```python
from build123d import *

# Parameters (mm, degrees)
PAD017_DEPTH                  = 15.3
PAD017_MIRRORED033_2_DEPTH    = 15.3
PAD023_DEPTH                  = 2
PAD023_MIRRORED043_2_DEPTH    = 2
SKETCH061_R                   = 1
PAD019_DEPTH                  = 4
POCKET060_DEPTH               = 6
POCKET060_MIRRORED038_2_DEPTH = 6
PAD020_DEPTH                  = 30
POCKET068_DEPTH               = 20
CHAMFER034_SIZE               = 1
CHAMFER026_SIZE               = 1
CHAMFER029_SIZE               = 0.5
CHAMFER028_SIZE               = 0.5
CHAMFER033_SIZE               = 0.5
POCKET063_DEPTH               = 5
SKETCH082_W                   = 9.4
SKETCH082_H                   = 50
POCKET066_DEPTH               = 5
POCKET053_DEPTH               = 10
POCKET065_DEPTH               = 10
POCKET052_DEPTH               = 10
POCKET056_DEPTH               = 10
POCKET057_DEPTH               = 10
POCKET071_DEPTH               = 10
SKETCH072_R                   = 2
POCKET072_DEPTH               = 5
CHAMFER031_SIZE               = 1.5


with BuildPart() as part:
    # Sketch076 → Pad017 (new body)
    with BuildSketch(Plane.XY):
        with BuildLine():
            ThreePointArc((-47.2, 25.2), (-49.32132, 24.32132), (-50.2, 22.2))
            Line((-50.2, 22.2), (-50.2, 0))
            Line((-52.2, 0), (-50.2, 0))
            Line((-52.2, 22.2), (-52.2, 0))
            ThreePointArc((-47.2, 27.2), (-50.735534, 25.735534), (-52.2, 22.2))
            Line((-47.2, 27.2), (0, 27.2))
            Line((0, 27.2), (0, 25.2))
            Line((-47.2, 25.2), (0, 25.2))
        make_face()
    pad017 = extrude(amount=PAD017_DEPTH)

    # Sketch076 Mirrored033 2 → Pad017 Mirrored033 2 (add)
    with BuildSketch(Plane(origin=(0, 0, 0), x_dir=(-1, 0, 0), z_dir=(0, 0, -1))):
        with BuildLine():
            ThreePointArc((-47.2, 25.2), (-49.32132, 24.32132), (-50.2, 22.2))
            Line((-50.2, 22.2), (-50.2, 0))
            Line((-52.2, 0), (-50.2, 0))
            Line((-52.2, 22.2), (-52.2, 0))
            ThreePointArc((-47.2, 27.2), (-50.735534, 25.735534), (-52.2, 22.2))
            Line((-47.2, 27.2), (0, 27.2))
            Line((0, 27.2), (0, 25.2))
            Line((-47.2, 25.2), (0, 25.2))
        make_face()
    pad017_mirrored033_2 = extrude(amount=-PAD017_MIRRORED033_2_DEPTH)

    # Mirrored031: Pad017, Pad017 Mirrored033 2 across Sketch076 H_Axis
    add(pad017.mirror(Plane.ZX))
    add(pad017_mirrored033_2.mirror(Plane.ZX))

    # Sketch074 → Pad023 (join)
    with BuildSketch(Plane.XY):
        with BuildLine():
            ThreePointArc((-47.2, 25.2), (-49.32132, 24.32132), (-50.2, 22.2))
            Line((-50.2, 22.2), (-50.2, 0))
            Line((-50.2, 0), (0, 0))
            Line((0, 0), (0, 25.2))
            Line((-47.2, 25.2), (0, 25.2))
        make_face()
    pad023 = extrude(amount=PAD023_DEPTH)

    # Sketch074 Mirrored043 2 → Pad023 Mirrored043 2 (add)
    with BuildSketch(Plane(origin=(0, 0, 0), x_dir=(-1, 0, 0), z_dir=(0, 0, -1))):
        with BuildLine():
            ThreePointArc((-47.2, 25.2), (-49.32132, 24.32132), (-50.2, 22.2))
            Line((-50.2, 22.2), (-50.2, 0))
            Line((-50.2, 0), (0, 0))
            Line((0, 0), (0, 25.2))
            Line((-47.2, 25.2), (0, 25.2))
        make_face()
    pad023_mirrored043_2 = extrude(amount=-PAD023_MIRRORED043_2_DEPTH)

    # Mirrored037: Pad023, Pad023 Mirrored043 2 across Sketch074 H_Axis
    add(pad023.mirror(Plane.ZX))
    add(pad023_mirrored043_2.mirror(Plane.ZX))

    # Sketch061 (on Face19 of MultiTransform012) → Pad019 (join)
    with BuildSketch(Plane.XY.offset(2)):
        with BuildLine():
            ThreePointArc((50.2, 22.2), (49.32132, 24.32132), (47.2, 25.2))
            Line((47.2, 25.2), (44, 25.2))
            Line((44, 22), (44, 25.2))
            ThreePointArc((44, 22), (44.87868, 19.87868), (47, 19))
            Line((47, 19), (50.2, 19))
            Line((50.2, 22.2), (50.2, 19))
        make_face()
        with Locations((47, 22)):
            Circle(SKETCH061_R, mode=Mode.SUBTRACT)
        with BuildLine():
            ThreePointArc((-41, 22), (-38, 19), (-35, 22))
            Line((-35, 22), (-35, 25.2))
            Line((-41, 25.2), (-35, 25.2))
            Line((-41, 22), (-41, 25.2))
        make_face()
        with Locations((-38, 22)):
            Circle(SKETCH061_R, mode=Mode.SUBTRACT)
    pad019 = extrude(amount=PAD019_DEPTH)

    # Mirrored035: Pad019 across Sketch061 H_Axis
    add(pad019.mirror(Plane(origin=(0, 0, 2), x_dir=(0, 0, 1), z_dir=(0, 1, 0))))

    # Sketch068 (on Face5 of Mirrored035) → Pocket060 (cut)
    with BuildSketch(Plane.XY.offset(15.3)):
        with BuildLine():
            ThreePointArc((-47.2, 27.2), (-50.735534, 25.735534), (-52.2, 22.2))
            Line((-52.2, 0), (-52.2, 22.2))
            Line((-51.1, 0), (-52.2, 0))
            Line((-51.1, 22.2), (-51.1, 0))
            ThreePointArc((-47.2, 26.1), (-49.957716, 24.957716), (-51.1, 22.2))
            Line((0, 26.1), (-47.2, 26.1))
            Line((0, 27.2), (0, 26.1))
            Line((-47.2, 27.2), (0, 27.2))
        make_face()
    pocket060 = extrude(amount=-POCKET060_DEPTH, mode=Mode.SUBTRACT)

    # Sketch068 Mirrored038 2 → Pocket060 Mirrored038 2 (cut)
    with BuildSketch(Plane(origin=(0, 0, 15.3), x_dir=(-1, 0, 0), z_dir=(0, 0, -1))):
        with BuildLine():
            ThreePointArc((-47.2, 27.2), (-50.735534, 25.735534), (-52.2, 22.2))
            Line((-52.2, 0), (-52.2, 22.2))
            Line((-51.1, 0), (-52.2, 0))
            Line((-51.1, 22.2), (-51.1, 0))
            ThreePointArc((-47.2, 26.1), (-49.957716, 24.957716), (-51.1, 22.2))
            Line((0, 26.1), (-47.2, 26.1))
            Line((0, 27.2), (0, 26.1))
            Line((-47.2, 27.2), (0, 27.2))
        make_face()
    pocket060_mirrored038_2 = extrude(amount=POCKET060_MIRRORED038_2_DEPTH, mode=Mode.SUBTRACT)

    # Mirrored042: Pocket060, Pocket060 Mirrored038 2 across Sketch068 H_Axis
    add(pocket060.mirror(Plane(origin=(0, 0, 15.3), x_dir=(0, 0, 1), z_dir=(0, 1, 0))), mode=Mode.SUBTRACT)
    add(pocket060_mirrored038_2.mirror(Plane(origin=(0, 0, 15.3), x_dir=(0, 0, 1), z_dir=(0, 1, 0))), mode=Mode.SUBTRACT)

    # Sketch060 → Pad020 (join, symmetric)
    with BuildSketch(Plane.YZ):
        with BuildLine():
            ThreePointArc((-26.1, 12.9), (-26.7, 12.3), (-26.1, 11.7))
            Line((-26.1, 12.9), (-26.1, 11.7))
        make_face()
    pad020 = extrude(amount=PAD020_DEPTH, both=True)

    # Sketch060 → Pocket068 (cut, symmetric)
    with BuildSketch(Plane.YZ):
        with BuildLine():
            ThreePointArc((-26.1, 12.9), (-26.7, 12.3), (-26.1, 11.7))
            Line((-26.1, 12.9), (-26.1, 11.7))
        make_face()
    pocket068 = extrude(amount=POCKET068_DEPTH, both=True, mode=Mode.SUBTRACT)

    # Mirrored034: Pad020, Pocket068 across Sketch060 V_Axis
    add(pad020.mirror(Plane(origin=(0, 0, 0), x_dir=(1, 0, 0), z_dir=(0, 1, 0))))
    add(pocket068.mirror(Plane(origin=(0, 0, 0), x_dir=(1, 0, 0), z_dir=(0, 1, 0))), mode=Mode.SUBTRACT)

    # Chamfer034
    chamfer034_edges = [part.edges().sort_by_distance(p)[0] for p in [
        (0, -27.2, 0),
    ]]
    chamfer(chamfer034_edges, length=CHAMFER034_SIZE)

    # Chamfer026
    chamfer026_edges = [part.edges().sort_by_distance(p)[0] for p in [
        (-35, 23.6, 6),
        (-35, -23.6, 6),
        (44, -23.6, 6),
        (44, 23.6, 6),
    ]]
    chamfer(chamfer026_edges, length=CHAMFER026_SIZE)

    # Chamfer029
    chamfer029_edges = [part.edges().sort_by_distance(p)[0] for p in [
        (-39, 22, 6),
        (46, 22, 6),
        (-39, -22, 6),
        (46, -22, 6),
    ]]
    chamfer(chamfer029_edges, length=CHAMFER029_SIZE)

    # Chamfer028
    chamfer028_edges = [part.edges().sort_by_distance(p)[0] for p in [
        (0, -26.1, 15.3),
    ]]
    chamfer(chamfer028_edges, length=CHAMFER028_SIZE)

    # Chamfer033
    chamfer033_edges = [part.edges().sort_by_distance(p)[0] for p in [
        (-23.6, -27.2, 9.3),
    ]]
    chamfer(chamfer033_edges, length=CHAMFER033_SIZE)

    # Sketch069 (on DatumPlane) → Pocket063 (cut)
    with BuildSketch(Plane.YZ.offset(52.2)):
        with BuildLine():
            ThreePointArc((7.9, 8.75), (8.266117, 7.866117), (9.15, 7.5))
            Line((9.15, 7.5), (15.85, 7.5))
            ThreePointArc((15.85, 7.5), (16.733883, 7.866117), (17.1, 8.75))
            Line((17.1, 8.75), (17.1, 58.75))
            Line((7.9, 58.75), (17.1, 58.75))
            Line((7.9, 8.75), (7.9, 58.75))
        make_face()
    extrude(amount=-POCKET063_DEPTH, mode=Mode.SUBTRACT)

    # Sketch082 (on DatumPlane) → Pocket066 (cut)
    with BuildSketch(Plane.YZ.offset(52.2)):
        with Locations((0, 32.6)):
            Rectangle(SKETCH082_W, SKETCH082_H)
    extrude(amount=-POCKET066_DEPTH, mode=Mode.SUBTRACT)

    # Sketch062 (on DatumPlane) → Pocket053 (cut)
    with BuildSketch(Plane.YZ.offset(52.2)):
        Polygon((-17.8, 7.6), (-7.2, 7.6), (-7.2, 15.6), (-12.1, 15.6), (-12.1, 18.1), (-14.1, 18.1), (-14.1, 15.6), (-17.8, 15.6), align=None)
    extrude(amount=-POCKET053_DEPTH, mode=Mode.SUBTRACT)

    # Sketch083 (on DatumPlane) → Pocket065 (cut)
    with BuildSketch(Plane(origin=(-52.2, 0, 0), x_dir=(0, -1, 0), z_dir=(-1, 0, 0))):
        Polygon((-25.62, 7.6), (-15.02, 7.6), (-15.02, 15.6), (-19.92, 15.6), (-19.92, 18.1), (-21.92, 18.1), (-21.92, 15.6), (-25.62, 15.6), align=None)
    extrude(amount=-POCKET065_DEPTH, mode=Mode.SUBTRACT)

    # Sketch063 (on DatumPlane) → Pocket052 (cut)
    with BuildSketch(Plane(origin=(-52.2, 0, 0), x_dir=(0, -1, 0), z_dir=(-1, 0, 0))):
        Polygon((-15.46, 7.6), (-4.86, 7.6), (-4.86, 15.6), (-9.76, 15.6), (-9.76, 18.1), (-11.76, 18.1), (-11.76, 15.6), (-15.46, 15.6), align=None)
    extrude(amount=-POCKET052_DEPTH, mode=Mode.SUBTRACT)

    # Sketch059 (on DatumPlane) → Pocket056 (cut)
    with BuildSketch(Plane(origin=(-52.2, 0, 0), x_dir=(0, -1, 0), z_dir=(-1, 0, 0))):
        Polygon((-5.3, 7.6), (5.3, 7.6), (5.3, 15.6), (0, 15.6), (0, 18.1), (-2, 18.1), (-2, 15.6), (-5.3, 15.6), align=None)
    extrude(amount=-POCKET056_DEPTH, mode=Mode.SUBTRACT)

    # Sketch071 (on DatumPlane) → Pocket057 (cut)
    with BuildSketch(Plane(origin=(-52.2, 0, 0), x_dir=(0, -1, 0), z_dir=(-1, 0, 0))):
        Polygon((4.86, 7.6), (15.46, 7.6), (15.46, 15.6), (10.56, 15.6), (10.56, 18.1), (8.56, 18.1), (8.56, 15.6), (4.86, 15.6), align=None)
    extrude(amount=-POCKET057_DEPTH, mode=Mode.SUBTRACT)

    # Sketch070 (on DatumPlane) → Pocket071 (cut)
    with BuildSketch(Plane(origin=(-52.2, 0, 0), x_dir=(0, -1, 0), z_dir=(-1, 0, 0))):
        Polygon((15.02, 7.6), (25.62, 7.6), (25.62, 15.6), (20.72, 15.6), (20.72, 18.1), (18.72, 18.1), (18.72, 15.6), (15.02, 15.6), align=None)
    extrude(amount=-POCKET071_DEPTH, mode=Mode.SUBTRACT)

    # Sketch072 (on DatumPlane) → Pocket072 (cut)
    with BuildSketch(Plane.XY.offset(2)):
        with Locations((-40, 15)):
            Circle(SKETCH072_R)
        with Locations((40, 15)):
            Circle(SKETCH072_R)
        with Locations((40, -15)):
            Circle(SKETCH072_R)
        with Locations((-40, -15)):
            Circle(SKETCH072_R)
    extrude(amount=-POCKET072_DEPTH, mode=Mode.SUBTRACT)

    # Chamfer031
    chamfer031_edges = [part.edges().sort_by_distance(p)[0] for p in [
        (-42, 15, 2),
        (38, 15, 2),
        (38, -15, 2),
        (-42, -15, 2),
    ]]
    chamfer(chamfer031_edges, length=CHAMFER031_SIZE)


solid = part.part
```
Model file for the job. Use its own axes, mm. A direction names the side the tool comes from. Round coordinates to 2 decimals unless told otherwise and drop trailing zeros. Write each loop counter-clockwise with the first axis right and the second up, starting at its lowest first coordinate (ties: lowest second). Pieces come first, ordered by that corner, then holes. Notation, with made-up numbers: (20, 23) - (27, 23) arc R6 cw to (27, 30) - close; hole circle Ø3 at (-34.75, 30.5). An arc over 180 degrees is marked (long way). Use CSV: the item, a comma, the result in double quotes. Start each with the question number.
Item 1: Two-plate mould, pull along Y, no slides. Class faces 4 (the face through (1, 27.2, 5)), 5 (the face through (50.8, -7.2, 10.5)), 6 (the face through (1, 0, 0)): released by +Y, released by -Y, zero draft, split by the parting line, or undercut.
Item 2: Band-saw the part on D-D (x = -5). Write the cut outline in (y, z), and give its area (3 significant figures).
Item 3: Band-saw the part on A-A (x = 40). State how many separate pieces and enclosed holes the cut face has, and give its area (3 significant figures).
Item 4: Pin check, flat tips, straight feed: P1, Ø1.5, axis at x = -7, z = 10.5, coming from the -Y side; P2, Ø4, axis at y = 2.5, z = 12, coming from the +X side; P3, Ø0.5, axis at y = -25.5, z = 11.5, coming from the -X side; P4, Ø0.7, axis at y = -26.5, z = 12.5, coming from the +X side. Stop position of each tip, or through.
Item 5: Band-saw the part on B-B (y = -15). Write the cut outline in (x, z), and give its area (3 significant figures).
Item 6: Drill centre lines: L1, parallel to X at y = -22, z = 4; L2, parallel to Y at x = -38, z = 2.8; L3, parallel to Y at x = 23, z = 3.75. Where is each one in solid material? Low to high. Write a range as [from, to].
Item 7: Tool access for faces 1 (the face through (50.8, 7.9, 12)), 2 (the face through (51.1, 6, 12)), 3 (the face through (48.14, -23.21, 6)): list every direction of +Z, -Z, +X, -X, +Y, -Y with a clear straight run to the whole face (end or side of a thin tool).
Item 8: Band-saw the part on C-C (x = -22). Write the cut outline in (y, z), and give its area (3 significant figures).
Checked values:
1,face 4,"released by +Y"
1,face 5,"undercut"
1,face 6,"zero draft"
2,outline,"(-27.2, 1) - (-26.2, 0) - (26.2, 0) - (27.2, 1) - (27.2, 8.8) - (26.7, 9.3) - (26.1, 9.3) - (26.1, 14.8) - (25.6, 15.3) - (25.2, 15.3) - (25.2, 2) - (-25.2, 2) - (-25.2, 15.3) - (-25.6, 15.3) - (-26.1, 14.8) - (-26.1, 9.3) - (-26.7, 9.3) - (-27.2, 8.8) - close"
2,area,"147 mm²"
3,separate pieces,"3"
3,enclosed holes,"0"
3,area,"127 mm²"
4,P1,"stops at y = -26.1"
4,P2,"passes through"
4,P3,"stops at x = -49.07"
4,P4,"stops at x = 30"
5,outline,"(-52.2, 1) - (-51.2, 0) - (-42, 0) - (-42, 0.5) - (-43.5, 2) - (-50.2, 2) - (-50.2, 7.6) - (-52.2, 7.6) - close; (-38, 0) - (38, 0) - (38, 0.5) - (36.5, 2) - (-36.5, 2) - (-38, 0.5) - close; (42, 0) - (51.2, 0) - (52.2, 1) - (52.2, 7.6) - (50.2, 7.6) - (50.2, 2) - (43.5, 2) - (42, 0.5) - close"
5,area,"210 mm²"
6,L1,"x = [-52.2, -50.2], [-41, -39], [-37, -35], [44, 46], [48, 52.2]"
6,L2,"y = [-27.2, -23], [-21, -19], [19, 21], [23, 27.2]"
6,L3,"y = [-27.2, -25.2], [25.2, 27.2]"
7,face 1,"+Z, +X, -X"
7,face 2,"+Z, +X, +Y, -Y"
7,face 3,"+Z"
8,outline,"(-27.2, 1) - (-26.2, 0) - (26.2, 0) - (27.2, 1) - (27.2, 8.8) - (26.7, 9.3) - (26.1, 9.3) - (26.1, 11.7) arc R0.6 ccw to (26.1, 12.9) - (26.1, 14.8) - (25.6, 15.3) - (25.2, 15.3) - (25.2, 2) - (-25.2, 2) - (-25.2, 15.3) - (-25.6, 15.3) - (-26.1, 14.8) - (-26.1, 12.9) arc R0.6 ccw to (-26.1, 11.7) - (-26.1, 9.3) - (-26.7, 9.3) - (-27.2, 8.8) - close"
8,area,"148 mm²"
